Model file for the job. Use its own axes, mm. A direction names the side the tool comes from. Give positions to 0.01 mm unless a question says otherwise; leave off trailing zeros. Write each loop counter-clockwise with the first axis right and the second up, starting at its lowest first coordinate (ties: lowest second). Pieces come first, ordered by that corner, then holes. Notation, with made-up numbers: (82, -20.75) - (110, -20.75) arc R7 cw to (110, -8.75) - close; hole circle Ø5 at (-23, 72). An arc over 180 degrees is marked (long way). One line per item, written item: value. Start each with the question number.
(1) Cut at D-D, the plane z = 17.25. List the corners of the cut face in (x, y).
(2) Cut at A-A, the plane y = 0. List the corners of the cut face in (x, z), and give its area (3 significant figures).
(3) Drop flat-ended pins along their axis: P1, Ø1, axis at y = 0, z = 8.5, coming from the +X side; P2, Ø2, axis at y = 0, z = 9, coming from the -X side; P3, Ø2, axis at x = 0, z = 9, coming from the +Y side. Give the stop position or say it passes through.
(4) 3-axis set-ups, long thin cutter, end or side, ignore diameter. For faces 1 (the face through (0, -15.2, 8)), 2 (the face through (0, 15.2, 8)), 3 (the face through (15.2, 0, 8)), 4 (the face through (-15.2, 0, 8)): which of +Z, -Z, +X, -X, +Y, -Y reach the whole face in a straight line?
(5) Probe L1, parallel to Z at x = 11.5, y = 11; L2, parallel to Y at x = 1, z = 22.5; L3, parallel to X at y = 0.5, z = 6. List the from-to ranges inside material, lowest first.
(6) Cut at C-C, the plane z = 9. List the corners of the cut face in (x, y), and give its area (3 significant figures).
Autodesk Fusion 360 part; units mm, degrees
sketch "End cap profile" plane through (0, 0, 0) normal (0, 1, 0) x (1, 0, 0)
  line L0 (0, 0) -> (21, 0)
  line L1 (21, 0) -> (21, -4)
  line L2 (21, -4) -> (14.7, -4)
  line L3 (14.7, -4) -> (14.7, -25.5)
  line L4 (14.7, -25.5) -> (12.2, -28)
  line L5 (12.2, -28) -> (0, -28)
  line L6 (0, -28) -> (0, 0)
  dimension "d76" = 21
  dimension "d77" = 4
  dimension "d78" = 14.7
  dimension "d79" = 28
  dimension "d80" = 2.5
  dimension "d81" = 2.5
revolve "End cap revolve" add sketch "End cap profile" angle 360 about axis through (0, 0, 1.75) along (0, 0, 1)
sketch "Crush rib" plane through (0, 0, 0) normal (0, 1, 0) x (1, 0, 0)
  line L0 (13.7, -5) -> (15.2, -5)
  line L1 (15.2, -5) -> (15.2, -11)
  line L2 (15.2, -11) -> (13.7, -26)
  line L3 (13.7, -26) -> (13.7, -5)
  dimension "d83" = 13.7
  dimension "d84" = 5
  dimension "d85" = 15.2
  dimension "d86" = 26
  dimension "d87" = 11
extrude "Crush rib (1)" add sketch "Crush rib" along normal mid plane 2
pattern_circular "Crush ribs" count 4 over 360 about axis through (0, 0, 1.75) along (0, 0, 1) of "Crush rib (1)"
equation "rodOuterDiameter = 33.4 mm"
equation "pipeInnerDiameter = 30.0 mm"
equation "endCapFlangeProud = 4.3 mm"
equation "endCapFlangeThickness = 4.0 mm"
equation "endCapStemLength = 24.0 mm"
equation "endCapStemDiameter = pipeInnerDiameter - 0.6 mm"
equation "endCapRibDiameter = pipeInnerDiameter + 0.4 mm"
equation "endCapTipChamfer = 2.5 mm"
equation "endCapRibWidth = 2.0 mm"
equation "endCapRibGripLength = 6.0 mm"
equation "d76 = rodOuterDiameter / 2 + endCapFlangeProud"
equation "d77 = endCapFlangeThickness"
equation "d78 = endCapStemDiameter / 2"
equation "d79 = endCapFlangeThickness + endCapStemLength"
equation "d80 = endCapTipChamfer"
equation "d81 = endCapTipChamfer"
equation "d83 = endCapStemDiameter / 2 - 1 mm"
equation "d84 = endCapFlangeThickness + 1 mm"
equation "d85 = endCapRibDiameter / 2"
equation "d86 = endCapFlangeThickness + endCapStemLength - 2 mm"
equation "d87 = endCapFlangeThickness + 1 mm + endCapRibGripLength"
equation "d88 = endCapRibWidth"
Answers follow:
1. outline: circle Ø29.4 at (0, 0)
2. outline: (-21, 0) - (21, 0) - (21, 4) - (14.7, 4) - (14.7, 5) - (15.2, 5) - (15.2, 11) - (14.7, 16) - (14.7, 25.5) - (12.2, 28) - (-12.2, 28) - (-14.7, 25.5) - (-14.7, 16) - (-15.2, 11) - (-15.2, 5) - (-14.7, 5) - (-14.7, 4) - (-21, 4) - close
2. area: 876 mm²
3. P1: stops at x = 15.2
3. P2: stops at x = -15.2
3. P3: stops at y = 15.2
4. face 1: +Z, +X, -X, -Y
4. face 2: +Z, +X, -X, +Y
4. face 3: +Z, +X, +Y, -Y
4. face 4: +Z, -X, +Y, -Y
5. L1: z = 0 to 4
5. L2: y = -14.67 to 14.67
5. L3: x = -15.2 to 15.2
6. outline: (-15.2, -1) - (-14.67, -1) arc R14.7 ccw to (-1, -14.67) - (-1, -15.2) - (1, -15.2) - (1, -14.67) arc R14.7 ccw to (14.67, -1) - (15.2, -1) - (15.2, 1) - (14.67, 1) arc R14.7 ccw to (1, 14.67) - (1, 15.2) - (-1, 15.2) - (-1, 14.67) arc R14.7 ccw to (-14.67, 1) - (-15.2, 1) - close
6. area: 683 mm²
